Input: part model. Units: mm. Frame: model coordinates. A direction names the side the tool comes from. Round coordinates to 2 decimals unless told otherwise and drop trailing zeros. Order: outer loops, then holes, each group sorted by start corner. A loop starts at its lowest first (then second) coordinate and runs counter-clockwise, first axis right, second up. Notation, with made-up numbers: (-5.5, -27.5) -> (29.5, -27.5) arc R22 ccw to (29.5, -8.5) -> close; hole circle Ø11 at (67, 70). An arc over 180 degrees is marked (long way). Use a Markdown table: item, result.
from build123d import *

# Parameters (mm, degrees)
BOSS_EXTRUDE1_DEPTH              = 330.2
BOSS_EXTRUDE1_DEPTH_BACK         = 330.2
SKETCH3_W                        = 50.8
SKETCH3_H                        = 25.4
SKETCH3_W_2                      = 44.45
SKETCH3_H_2                      = 19.05
F_1_4_0_25_DIAMETER_HOLE3_D      = 6.35
F_1_4_0_25_DIAMETER_HOLE4_D      = 6.35
F_1_4_0_25_DIAMETER_HOLE5_D      = 6.35
F_1_4_0_25_DIAMETER_HOLE6_D      = 6.35
F_1_4_0_25_DIAMETER_HOLE7_D      = 6.35
F_1_4_0_25_DIAMETER_HOLE8_D      = 6.35
F_13_64_0_20313_DIAMETER_HOLE1_D = 5.159502
F_1_2_0_5_DIAMETER_HOLE1_D       = 12.7
F_1_2_0_5_DIAMETER_HOLE1_DEPTH   = 6.35
F_1_2_0_5_DIAMETER_HOLE1_TIP     = 3.815464931
F_10_CLEARANCE_HOLE1_AT_2_COUNT  = 2
F_10_CLEARANCE_HOLE1_AT_2_PITCH  = 25.4
F_10_CLEARANCE_HOLE1_AT_3_COUNT  = 2
F_10_CLEARANCE_HOLE1_AT_3_PITCH  = 160.769159045
F_10_CLEARANCE_HOLE1_AT_4_COUNT  = 2
F_10_CLEARANCE_HOLE1_AT_4_PITCH  = 158.75


with BuildPart() as part:
    # Sketch3 → Boss-Extrude1 (new, two sides: drawn at the far end of the back side and taken through both)
    with BuildSketch(Plane.XY.offset(-BOSS_EXTRUDE1_DEPTH_BACK)):
        Rectangle(SKETCH3_W, SKETCH3_H)
        Rectangle(SKETCH3_W_2, SKETCH3_H_2, mode=Mode.SUBTRACT)
    extrude(amount=BOSS_EXTRUDE1_DEPTH + BOSS_EXTRUDE1_DEPTH_BACK)

    # 1/4 (0.25) Diameter Hole3 (through all)
    with Locations(Plane.ZY.offset(25.4)):
        with Locations((-317.5, 0)):
            Hole(F_1_4_0_25_DIAMETER_HOLE3_D / 2)

    # 1/4 (0.25) Diameter Hole4 (through all)
    with Locations(Plane.ZY.offset(25.4)):
        with Locations((292.1, 0), (317.5, 0)):
            Hole(F_1_4_0_25_DIAMETER_HOLE4_D / 2)

    # 1/4 (0.25) Diameter Hole5 (through all)
    with Locations(Plane(origin=(25.4, 0, 0), x_dir=(0, 0, -1), z_dir=(1, 0, 0))):
        with Locations((292.1, 0), (266.7, 0)):
            Hole(F_1_4_0_25_DIAMETER_HOLE5_D / 2)

    # 1/4 (0.25) Diameter Hole6 (through all)
    with Locations(Plane(origin=(25.4, 0, 0), x_dir=(0, 0, -1), z_dir=(1, 0, 0))):
        with Locations((215.9, 0), (241.3, 0)):
            Hole(F_1_4_0_25_DIAMETER_HOLE6_D / 2)

    # 1/4 (0.25) Diameter Hole7 (through all)
    with Locations(Plane(origin=(25.4, 0, 0), x_dir=(0, 0, -1), z_dir=(1, 0, 0))):
        with Locations((-190.5, 0), (-215.9, 0)):
            Hole(F_1_4_0_25_DIAMETER_HOLE7_D / 2)

    # 1/4 (0.25) Diameter Hole8 (through all)
    with Locations(Plane(origin=(25.4, 0, 0), x_dir=(0, 0, -1), z_dir=(1, 0, 0))):
        with Locations((-266.7, 0), (-241.3, 0)):
            Hole(F_1_4_0_25_DIAMETER_HOLE8_D / 2)

    # 13/64 (0.20313) Diameter Hole1 (through all)
    with Locations(Plane(origin=(25.4, 0, 0), x_dir=(0, 0, -1), z_dir=(1, 0, 0))):
        with Locations((-152.4, 0), (177.8, 0)):
            Hole(F_13_64_0_20313_DIAMETER_HOLE1_D / 2)

    # 1/2 (0.5) Diameter Hole1
    with Locations(Plane.ZY.offset(25.4)):
        with Locations((-146.050000508, 4.9e-08), (120.65, 1.7e-08)):
            Hole(F_1_2_0_5_DIAMETER_HOLE1_D / 2, depth=F_1_2_0_5_DIAMETER_HOLE1_DEPTH)
            with Locations((0, 0, -(F_1_2_0_5_DIAMETER_HOLE1_DEPTH + F_1_2_0_5_DIAMETER_HOLE1_TIP / 2))):  # 118° drill point
                Cone(0, F_1_2_0_5_DIAMETER_HOLE1_D / 2, F_1_2_0_5_DIAMETER_HOLE1_TIP, mode=Mode.SUBTRACT)

    # Sketch39 → #10 Clearance Hole1 (revolve, cut)
    with BuildSketch(Plane(origin=(-7.747762, -12.7, -30.0312328), x_dir=(0, 0, -1), z_dir=(1, 0, 0))):
        Polygon((0, 0), (0, 25.4), (5.2197, 25.4), (2.4892, 22.258919064), (2.4892, 0), align=None)
    f_10_clearance_hole1 = revolve(axis=Axis((-7.747762, -19.05, -30.0312328), (0, 1, 0)), mode=Mode.SUBTRACT)

    # #10 Clearance Hole1 at 2: #10 Clearance Hole1 ×2
    with Locations(*[(i * F_10_CLEARANCE_HOLE1_AT_2_PITCH, 0, 0) for i in range(1, F_10_CLEARANCE_HOLE1_AT_2_COUNT)]):
        add(f_10_clearance_hole1, mode=Mode.SUBTRACT)

    # #10 Clearance Hole1 at 3: #10 Clearance Hole1 ×2
    with Locations(*[Vector(0.15799050110667284, 0, 0.9874406319167054) * (i * F_10_CLEARANCE_HOLE1_AT_3_PITCH) for i in range(1, F_10_CLEARANCE_HOLE1_AT_3_COUNT)]):
        add(f_10_clearance_hole1, mode=Mode.SUBTRACT)

    # #10 Clearance Hole1 at 4: #10 Clearance Hole1 ×2
    with Locations(*[(0, 0, i * F_10_CLEARANCE_HOLE1_AT_4_PITCH) for i in range(1, F_10_CLEARANCE_HOLE1_AT_4_COUNT)]):
        add(f_10_clearance_hole1, mode=Mode.SUBTRACT)


solid = part.part
1) Cut plane A-A on z = -146.05. Return loops of the section in (x, y) (3 decimals), and give its area (3 significant figures).
Answer key:
| item | result |
|---|---|
| outline | (-25.4, -12.7) -> (25.4, -12.7) -> (25.4, 12.7) -> (-25.4, 12.7) -> (-25.4, 6.35) -> (-22.225, 6.35) -> (-22.225, 9.525) -> (22.225, 9.525) -> (22.225, -9.525) -> (-22.225, -9.525) -> (-22.225, -6.35) -> (-25.4, -6.35) -> close |
| area | 403 mm^2 |
2) Contact query for flat-ended pins moving along their axis: P1, Ø8, axis at x = 17.65, z = 128.72, coming from the +Y side; P2, Ø5.5, axis at x = -7.75, z = -30.03, coming from the +Y side. Output: stop coordinate, or through.
Answer key:
| item | result |
|---|---|
| P1 | stops at y = 11.3 |
| P2 | stops at y = 9.86 |
3) Set-up query: faces 1 (the face through (0, -12.7, -5)), 2 (the face through (22.225, 0, -5)), 3 (the face through (-23.79, 1.907, -152.107)). Return all of +Z, -Z, +X, -X, +Y, -Y with unobstructed straight access to the full face (end or side cutting, diameter ignored); none if empty.
Answer key:
| item | result |
|---|---|
| face 1 | +Z, -Z, +X, -X, -Y |
| face 2 | +Z, -Z |
| face 3 | -X |
4) Ray query, probe 1 along X at (y, z) = (-4.5, 43) (3 decimals); probe 2 along Y at (x, z) = (4, -40.5) (3 decimals); probe 3 along Y at (x, z) = (24.15, 266.7) (3 decimals). Return the intervals inside material, ascending.
Answer key:
| item | result |
|---|---|
| probe 1 | x = -25.4 to -22.225, 22.225 to 25.4 |
| probe 2 | y = -12.7 to -9.525, 9.525 to 12.7 |
| probe 3 | y = -12.7 to -3.175, 3.175 to 12.7 |
5) Cut plane B-B on z = -14.5. Return loops of the section in (x, y) (3 decimals).
Answer key:
| item | result |
|---|---|
| outline | (-25.4, -12.7) -> (25.4, -12.7) -> (25.4, 12.7) -> (-25.4, 12.7) -> close; hole (-22.225, -9.525) -> (22.225, -9.525) -> (22.225, 9.525) -> (-22.225, 9.525) -> close |
6) Draft query along Z for faces 4 (the face through (0, 10, 330.2)), 5 (the face through (-10.347, 9.711, -29.69)), 6 (the face through (-22.225, 0, -5)). Return one class per face: released by +Z, released by -Z, zero draft, split by the parting line, or undercut.
Answer key:
| item | result |
|---|---|
| face 4 | released by +Z |
| face 5 | undercut |
| face 6 | zero draft |
